Geometry: final body of the model. Coordinates: model frame, mm. Face numbers are marked on the shaded views. A direction names the side the tool comes from. Give positions to 0.01 mm unless a question says otherwise; leave off trailing zeros. Write each loop counter-clockwise with the first axis right and the second up, starting at its lowest first coordinate (ties: lowest second). Pieces come first, ordered by that corner, then holes. Notation, with made-up numbers: (61, 78.5) -> (113, 78.5) arc R28 ccw to (113, 107.5) -> close; hole circle Ø8 at (37.25, 14.25). An arc over 180 degrees is marked (long way). Answer as a JSON object with one key per item and string values. Group by question number.
(1) Section query A-A on x = 0. Output: boundary loops of the cut face in (y, z).
(2) Contact query for flat-ended pins moving along their axis: pin 1 Ø3 at (y, z) = (-26, -17.5) entering from -X; pin 2 Ø1.5 at (y, z) = (-7.5, -38.5) entering from -X; pin 3 Ø6 at (x, y) = (23, -30) entering from -Z. Output: stop coordinate, or through.
(3) Set-up query: the marked faces 1 and 2. Return all of +Z, -Z, +X, -X, +Y, -Y with unobstructed straight access to the full face (end or side cutting, diameter ignored); none if empty.
(4) Section query C-C on y = -13. Output: boundary loops of the cut face in (x, z).
(5) Draft query along X for the marked faces 3, 4 and 5. Return one class per face: +X half, -X half, draft (parallel to the pull), parting line (faces both ways), or undercut.
(6) Material intervals for probe 1 along X at (y, z) = (17, 0); probe 2 along Y at (x, z) = (61, -35.5); probe 3 along X at (y, z) = (6.5, -5), sorted ascending.
(7) Section query D-D on x = 46. Output: boundary loops of the cut face in (y, z), plus the area to 3 significant figures.
(8) Section query B-B on z = 0. Output: boundary loops of the cut face in (x, y).
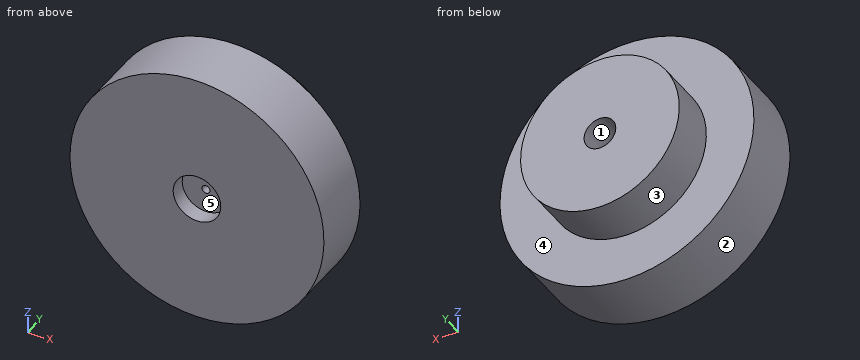
from build123d import *

# Parameters (mm, degrees)
HOLE_WIZARD_M6_2_D = 5


with BuildPart() as part:
    # 草图1 → 旋转1 (revolve)
    with BuildSketch(Plane.XY, mode=Mode.PRIVATE) as revolve_1_sk:
        Polygon((10, 30), (50, 30), (50, 0), (80, 0), (80, -40), (33.191510013, -40), (15, -40), (15, -30), (0, -30), (0, 0), (10, 0), align=None)
    revolve(revolve_1_sk.sketch.rotate(Axis((0, -30, 0), (0, 1, 0)), 90), axis=Axis((0, -30, 0), (0, 1, 0)))

    # M6 螺纹孔2 (through all)
    with Locations(Plane(origin=(0, -30, 0), x_dir=(-1, 0, 0), z_dir=(0, -1, 0))):
        with Locations((0, 0)):
            Hole(HOLE_WIZARD_M6_2_D / 2)


solid = part.part
Answer list:
{
 "1": {"outline": "(-40, -80) -> (0, -80) -> (0, -50) -> (30, -50) -> (30, -10) -> (0, -10) -> (0, -2.5) -> (-30, -2.5) -> (-30, -15) -> (-40, -15) -> close; (-40, 15) -> (-30, 15) -> (-30, 2.5) -> (0, 2.5) -> (0, 10) -> (30, 10) -> (30, 50) -> (0, 50) -> (0, 80) -> (-40, 80) -> close"},
 "2": {"pin 1": "x = -78.38", "pin 2": "x = -70.53", "pin 3": "z = -77.46"},
 "3": {"face 1": "+Y", "face 2": "+Y, -Y"},
 "4": {"outline": "circle Ø160 at (0, 0); hole circle Ø5 at (0, 0)"},
 "5": {"face 3": "parting line", "face 4": "draft", "face 5": "undercut"},
 "6": {"probe 1": "-50 to -10, 10 to 50", "probe 2": "-40 to 0", "probe 3": "-49.75 to -8.66, 8.66 to 49.75"},
 "7": {"outline": "(-40, -65.45) -> (0, -65.45) -> (0, -19.6) -> (30, -19.6) -> (30, 19.6) -> (0, 19.6) -> (0, 65.45) -> (-40, 65.45) -> close", "area": "6,410 mm2"},
 "8": {"outline": "(-80, -40) -> (-15, -40) -> (-15, -30) -> (-2.5, -30) -> (-2.5, 0) -> (-10, 0) -> (-10, 30) -> (-50, 30) -> (-50, 0) -> (-80, 0) -> close; (2.5, -30) -> (15, -30) -> (15, -40) -> (80, -40) -> (80, 0) -> (50, 0) -> (50, 30) -> (10, 30) -> (10, 0) -> (2.5, 0) -> close"}
}
